Here's how the part is built. I have some questions about the finished solid (model axes, mm). A direction names the side the tool comes from. Coordinates: 2 decimals unless noted, no trailing zeros. Write each loop counter-clockwise with the first axis right and the second up, starting at its lowest first coordinate (ties: lowest second). Pieces come first, ordered by that corner, then holes.
(1) Imagine slicing it at C-C, the plane z = 3. State how many separate pieces and enclosed holes the cut face has, plus the area to 3 significant figures.
(2) Which directions (+Z, -Z, +X, -X, +Y, -Y) give clear straight access to the entire face, cutting with the end or side of a thin tool? Please do faces 5 (the cylindrical face through (91, 33, 4)), 6 (the flat face through (80, 22, 4)).
(3) Thinking about a two-plate mould opening in Y: for faces 1 (the flat face through (52, 0, 4)), 2 (the flat face through (42, 9, 7)), 3 (the flat face through (92, 17, 4)), 4 (the cylindrical face through (42, 27, 2)), which applies, released by +Y, released by -Y, zero draft, split by the parting line, or undercut?
(4) Imagine slicing it at D-D, the plane y = 28. List the corners of the cut face in (x, z) for me.
(5) Imagine slicing it at B-B, the plane x = 42. List the corners of the cut face in (y, z) for me.
(6) Please list where these lines run through material, in increasing order: probe 1 along Y at (x, z) = (17.5, 5.75); probe 2 along X at (y, z) = (9.5, 5.5); probe 3 along Y at (x, z) = (61, 6).
(7) For pin 1 Ø2 at (y, z) = (11, 5) entering from -X, with a flat end and sliding along its axis, tell me the tip position at first contact or that it passes through.
(8) Imagine slicing it at A-A, the plane y = 20.5. List the corners of the cut face in (x, z) for me, plus the area to 3 significant figures.
```python
from build123d import *

# Parameters (mm, degrees)
F0_R     = 12.5
F1_DEPTH = 8


with BuildPart() as f1:
    # F0 (on Top) → F1 (new body)
    with BuildSketch(Plane.XY):
        with BuildLine():
            ThreePointArc((0, 17.5), (5.125631, 5.125631), (17.5, 0))
            Line((17.5, 0), (87, 0))
            ThreePointArc((87, 0), (90.535534, 1.464466), (92, 5))
            Line((92, 5), (92, 30))
            ThreePointArc((92, 30), (90.535534, 33.535534), (87, 35))
            Line((87, 35), (17.5, 35))
            ThreePointArc((17.5, 35), (5.125631, 29.874369), (0, 17.5))
        make_face()
        with Locations((17.5, 17.5)):
            Circle(F0_R, mode=Mode.SUBTRACT)
    extrude(amount=F1_DEPTH)

    # F2 (on face) → F3 (revolve, cut)
    with BuildSketch(Plane.XY.offset(8)):
        Polygon((42, 22), (42, 9), (45.5, 9), (45.5, 22), (49, 22), (49, 24), (48, 24), (48, 29), (42, 29), (42, 24), align=None)
    revolve(axis=Axis((42, 15.5, 8), (0, 1, 0)), mode=Mode.SUBTRACT)

    # F2 (on face) → F4 (revolve, cut)
    with BuildSketch(Plane.XY.offset(8)):
        Polygon((61, 22), (61, 9), (64.5, 9), (64.5, 22), (68, 22), (68, 24), (67, 24), (67, 29), (61, 29), (61, 24), align=None)
    revolve(axis=Axis((61, 15.5, 8), (0, 1, 0)), mode=Mode.SUBTRACT)

    # F2 (on face) → F5 (revolve, cut)
    with BuildSketch(Plane.XY.offset(8)):
        Polygon((80, 22), (80, 9), (83.5, 9), (83.5, 22), (87, 22), (87, 24), (86, 24), (86, 29), (80, 29), (80, 24), align=None)
    revolve(axis=Axis((80, 15.5, 8), (0, 1, 0)), mode=Mode.SUBTRACT)


solid = f1.part
```
Recorded:
1. separate pieces: 1
1. enclosed holes: 4
1. area: 2,430 mm2
2. face 5: +Z, -Z, +X, +Y
2. face 6: +Z
3. face 1: released by -Y
3. face 2: undercut
3. face 3: zero draft
3. face 4: undercut
4. outline: (3.5, 0) - (10.72, 0) - (10.72, 8) - (3.5, 8) - close; (24.28, 0) - (92, 0) - (92, 8) - (86, 8) arc R6 cw to (74, 8) - (67, 8) arc R6 cw to (55, 8) - (48, 8) arc R6 cw to (36, 8) - (24.28, 8) - close
5. outline: (0, 0) - (35, 0) - (35, 8) - (29, 8) - (29, 2) - (24, 2) - (24, 1) - (22, 1) - (22, 4.5) - (9, 4.5) - (9, 8) - (0, 8) - close
6. probe 1: y = 0 to 5, 30 to 35
6. probe 2: x = 1.94 to 7.9, 27.1 to 39.55, 44.45 to 58.55, 63.45 to 77.55, 82.45 to 92
6. probe 3: y = 0 to 9, 29 to 35
7. pin 1: stops at x = 0.89
8. outline: (0.26, 0) - (5.37, 0) - (5.37, 8) - (0.26, 8) - close; (29.63, 0) - (92, 0) - (92, 8) - (83.5, 8) arc R3.5 cw to (76.5, 8) - (64.5, 8) arc R3.5 cw to (57.5, 8) - (45.5, 8) arc R3.5 cw to (38.5, 8) - (29.63, 8) - close
8. area: 482 mm2
